Check sheet for the modelled part. Datum: model origin and axes. Units: mm. Face numbers are marked on the shaded views. A direction names the side the tool comes from. Coordinates: 2 decimals unless noted, no trailing zeros. Write each loop counter-clockwise with the first axis right and the second up, starting at its lowest first coordinate (ties: lowest second). Pieces come first, ordered by that corner, then holes. Notation, with made-up numbers: M 75,67.25 L 94,67.25 A19 cw 94,79.25 Z; hole C 88.25,-18.5 d1. An arc over 180 degrees is marked long. Answer as CSV lines item,"result". Start each with the question number.
Q1. Sectioned sample at A-A, the plane z = 171. Record the cut outline in (x, y), then the cut area to 3 significant figures.
Q2. Thickness scan on line 1 along X through (y, z) = (5, 43.5); line 2 along Z through (x, y) = (40, 6.5); line 3 along X through (y, z) = (-1, 42.5). Record the ranges inside material, lowest first. Write a range as from..to.
Q3. Mould release check, pull along Y, two halves, no side actions. Record for the marked faces 4, 5 and 6: pulls with the +Y half, pulls with the -Y half, needs draft (parallel to the pull), parting line crosses it, or undercut.
Q4. Depth check by flat-ended pin: pin 1 Ø12 at (y, z) = (-44.5, 65) entering from -X; pin 2 Ø4 at (y, z) = (-40.5, 32) entering from -X; pin 3 Ø1.5 at (x, y) = (-58.5, -39.5) entering from -Z. Enter the tip coordinate at first touch or a pass-through.
Q5. Access from +Z, -Z, +X, -X, +Y, -Y to the whole of each face (thin tool, end or side, straight path). Record for the marked faces 1, 2 and 3.
Q6. Sectioned sample at D-D, the plane z = 112. Record the cut outline in (x, y), then the cut area to 3 significant figures.
Q7. Sectioned sample at C-C, the plane x = 67.5. Record the cut outline in (y, z), then the cut area to 3 significant figures.
Q8. Sectioned sample at B-B, the plane y = 12. Record the cut outline in (x, z).
from build123d import *

# Parameters (mm, degrees)
F2_T      = -2.54
F3_W      = 25.4
F3_H      = 254
F4_DEPTH  = 38.1
F7_DEPTH  = 25.4
F12_DEPTH = 1.27
F14_W     = 304.8
F14_H     = 76.2
F15_DEPTH = 5.08


with BuildPart() as f1:
    # F0 (on Front) → F1 (revolve)
    with BuildSketch(Plane.XZ):
        with BuildLine():
            Line((25.4, 0), (0, 0))
            Line((0, 0), (0, -12.7))
            ThreePointArc((0, -12.7), (14.1990316571, -9.3480633142), (25.4, 0))
        make_face()
    revolve(axis=Axis((0, 0, -6.35), (0, 0, -1)))

    # F2
    f2_openings = [f1.faces().sort_by_distance(p)[0] for p in [
        (0, 0, 0),
    ]]
    offset(amount=F2_T, openings=f2_openings)



with BuildPart() as f4:
    # F3 (on Front) → F4 (new body, symmetric)
    with BuildSketch(Plane.XZ):
        with Locations((139.7, 63.5)):
            Rectangle(F3_W, F3_H)
    extrude(amount=F4_DEPTH, both=True)


with BuildPart() as f5_1:
    # F5: instance of F4
    add(f4.part.mirror(Plane.YZ))


with BuildPart() as f7:
    # F6 (on face) → F7 (new body)
    with BuildSketch(Plane.XZ.offset(38.1)):
        Polygon((147.8155081967, 165.5213901639), (127, 190.5), (-147.8256681967, -38.5213901639), (-127.01016, -63.5), align=None)
    extrude(amount=F7_DEPTH)


with BuildPart() as f8_1:
    # F8: instance of F7
    add(f7.part.mirror(Plane.XZ))


with BuildPart() as f9_1:
    # F9: instance of F8_1
    add(f8_1.part.mirror(Plane.YZ))


with BuildPart() as f12:
    # F11 (on Front) → F12 (new body, symmetric)
    with BuildSketch(Plane.XZ):
        Polygon((-22.86, 0), (-127, 190.5), (-127, 185.8536585366), (-25.4, 0), align=None)
    extrude(amount=F12_DEPTH, both=True)


with BuildPart() as f13_1:
    # F13: instance of F12
    add(f12.part.mirror(Plane.YZ))


with BuildPart() as f1_1:
    add(f1.part)

    add(f4.part)  # F15 merges F4

    add(f5_1.part)  # F15 merges F5_1

    add(f7.part)  # F15 merges F7

    add(f9_1.part)  # F15 merges F9_1

    add(f12.part)  # F15 merges F12

    add(f13_1.part)  # F15 merges F13_1
    # F14 (on face) → F15 (join)
    with BuildSketch(Plane(origin=(0, 0, -63.5), x_dir=(1, 0, 0), z_dir=(0, 0, -1))):
        Rectangle(F14_W, F14_H)
    extrude(amount=F15_DEPTH)


solid = f1_1.part
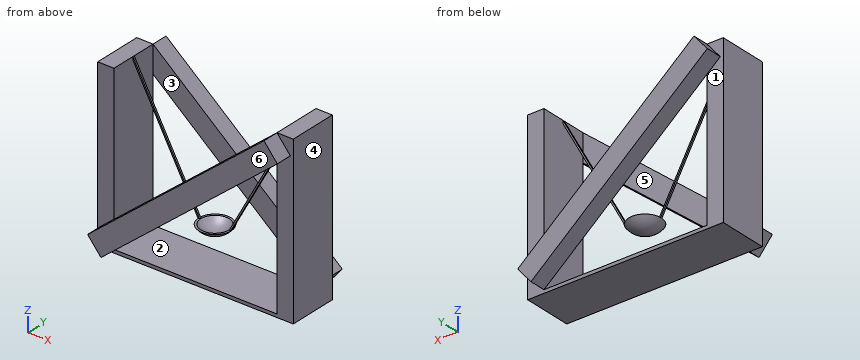
Output:
1,outline,"M -152.4,-38.1 L -127,-38.1 L -127,38.1 L -103.6,38.1 L -103.6,63.5 L -143.25,63.5 L -143.25,38.1 L -152.4,38.1 Z; M -118.88,-1.27 L -116.34,-1.27 L -116.34,1.27 L -118.88,1.27 Z; M 103.6,-63.5 L 143.25,-63.5 L 143.25,-38.1 L 152.4,-38.1 L 152.4,38.1 L 127,38.1 L 127,-38.1 L 103.6,-38.1 Z; M 116.34,-1.27 L 118.88,-1.27 L 118.88,1.27 L 116.34,1.27 Z"
1,area,"5,900 mm^2"
2,line 1,"x = -152.4..-127, 127..152.4"
2,line 2,"z = -68.58..-63.5"
2,line 3,"x = -152.4..-127, -48.63..-46.09, 46.09..48.63, 127..152.4"
3,face 4,"needs draft"
3,face 5,"undercut"
3,face 6,"pulls with the -Y half"
4,pin 1,"stops at x = -30.8"
4,pin 2,"stops at x = -65.6"
4,pin 3,"stops at z = -7.03"
5,face 1,"+Y"
5,face 2,"+Y, -Y"
5,face 3,"+Z"
6,outline,"M -152.4,-38.1 L -127,-38.1 L -127,38.1 L -152.4,38.1 Z; M -86.63,-1.27 L -84.09,-1.27 L -84.09,1.27 L -86.63,1.27 Z; M -83.59,38.1 L -32.8,38.1 L -32.8,63.5 L -83.59,63.5 Z; M 32.8,-63.5 L 83.59,-63.5 L 83.59,-38.1 L 32.8,-38.1 Z; M 84.09,-1.27 L 86.63,-1.27 L 86.63,1.27 L 84.09,1.27 Z; M 127,-38.1 L 152.4,-38.1 L 152.4,38.1 L 127,38.1 Z"
6,area,"6,460 mm^2"
7,outline,"M -63.5,98.59 L -38.1,98.59 L -38.1,140.92 L -63.5,140.92 Z; M -38.1,-68.58 L 38.1,-68.58 L 38.1,-63.5 L -38.1,-63.5 Z; M -1.27,77.01 L 1.27,77.01 L 1.27,81.66 L -1.27,81.66 Z; M 38.1,-13.91 L 63.5,-13.91 L 63.5,28.42 L 38.1,28.42 Z"
7,area,"2,550 mm^2"
8,outline,"M -152.4,-68.58 L 152.4,-68.58 L 152.4,190.5 L 127,190.5 L 127,-63.5 L -127,-63.5 L -127,190.5 L -152.4,190.5 Z; M -22.39,0 A29.39 ccw 22.39,0 L 18.61,0 A26.63 cw -18.61,0 Z"
